Could you check a few things on this model? Use its own coordinates, in mm. A direction names the side the tool comes from. Round coordinates to 2 decimals unless told otherwise and drop trailing zeros. Write each loop counter-clockwise with the first axis right and the second up, starting at its lowest first coordinate (ties: lowest second). Pieces come first, ordered by that corner, then holes. Notation, with made-up numbers: (-16.75, 26) -> (-2.75, 26) arc R28 ccw to (-2.75, 63) -> close; hole circle Ø11 at (40.5, 61). An arc over 180 degrees is marked (long way). Return JSON: item names as keys, results as strings.
from build123d import *

# Parameters (mm, degrees)
SKETCH_1_W          = 10
SKETCH_1_H          = 10
SKETCH_1_W_2        = 8
SKETCH_1_H_2        = 8
EXTRUDE_1_DEPTH     = 495
SKETCH_2_R          = 1.6
CUT_EXTRUDE_1_DEPTH = 496.126246527
CUT_EXTRUDE_2_REACH = 497.126
SKETCH_3_R          = 3
SKETCH_8_R          = 1.6
CUT_EXTRUDE_7_DEPTH = 496.126246527


with BuildPart() as part:
    # ｽｹｯﾁ1 → 押し出し-薄板1 (new body)
    with BuildSketch(Plane.XY):
        Rectangle(SKETCH_1_W, SKETCH_1_H)
        Rectangle(SKETCH_1_W_2, SKETCH_1_H_2, mode=Mode.SUBTRACT)
    extrude(amount=EXTRUDE_1_DEPTH)

    # ｽｹｯﾁ2 → ｶｯﾄ - 押し出し1 (cut, through all)
    with BuildSketch(Plane(origin=(0, 5, 0), x_dir=(1, 0, 0), z_dir=(0, 1, 0))):
        with Locations(Location((0, -5, 0), (0, 0, 180))):
            Circle(SKETCH_2_R)
        with Locations(Location((0, -490, 0), (0, 0, 180))):
            Circle(SKETCH_2_R)
        with Locations(Location((0, -470, 0), (0, 0, 180))):
            Circle(SKETCH_2_R)
    extrude(amount=-CUT_EXTRUDE_1_DEPTH, mode=Mode.SUBTRACT)

    # ｽｹｯﾁ3 → ｶｯﾄ - 押し出し2 (cut, up to next)
    with BuildSketch(Plane(origin=(0, 5, 0), x_dir=(1, 0, 0), z_dir=(0, 1, 0)), mode=Mode.PRIVATE) as cut_extrude_2_sk1:
        with Locations(Location((0, -5, 0), (0, 0, 180))):
            Circle(SKETCH_3_R)
    cut_extrude_2_tool1 = extrude(cut_extrude_2_sk1.sketch, amount=-CUT_EXTRUDE_2_REACH, mode=Mode.PRIVATE) & part.part
    # ｽｹｯﾁ3 → ｶｯﾄ - 押し出し2 (cut, up to next)
    with BuildSketch(Plane(origin=(0, 5, 0), x_dir=(1, 0, 0), z_dir=(0, 1, 0)), mode=Mode.PRIVATE) as cut_extrude_2_sk2:
        with Locations(Location((0, -490, 0), (0, 0, 180))):
            Circle(SKETCH_3_R)
    cut_extrude_2_tool2 = extrude(cut_extrude_2_sk2.sketch, amount=-CUT_EXTRUDE_2_REACH, mode=Mode.PRIVATE) & part.part
    # ｽｹｯﾁ3 → ｶｯﾄ - 押し出し2 (cut, up to next)
    with BuildSketch(Plane(origin=(0, 5, 0), x_dir=(1, 0, 0), z_dir=(0, 1, 0)), mode=Mode.PRIVATE) as cut_extrude_2_sk3:
        with Locations(Location((0, -470, 0), (0, 0, 180))):
            Circle(SKETCH_3_R)
    cut_extrude_2_tool3 = extrude(cut_extrude_2_sk3.sketch, amount=-CUT_EXTRUDE_2_REACH, mode=Mode.PRIVATE) & part.part
    add(cut_extrude_2_tool1.solids().sort_by_distance((0, 5, 5))[0], mode=Mode.SUBTRACT)
    add(cut_extrude_2_tool2.solids().sort_by_distance((0, 5, 490))[0], mode=Mode.SUBTRACT)
    add(cut_extrude_2_tool3.solids().sort_by_distance((0, 5, 470))[0], mode=Mode.SUBTRACT)

    # ｽｹｯﾁ8 → ｶｯﾄ - 押し出し7 (cut, through all)
    with BuildSketch(Plane(origin=(5, 0, 0), x_dir=(0, 0, -1), z_dir=(1, 0, 0))):
        with Locations(Location((-490, 0, 0), (0, 0, 90))):
            Circle(SKETCH_8_R)
        with Locations(Location((-475, 0, 0), (0, 0, 90))):
            Circle(SKETCH_8_R)
    extrude(amount=-CUT_EXTRUDE_7_DEPTH, mode=Mode.SUBTRACT)


solid = part.part
1) I want a section at A-A, the plane y = 0. Please give me the cut outline in (x, z).
Return value:
{"outline": "(-5, 0) -> (-4, 0) -> (-4, 473.4) -> (-5, 473.4) -> close; (-5, 476.6) -> (-4, 476.6) -> (-4, 488.4) -> (-5, 488.4) -> close; (-5, 491.6) -> (-4, 491.6) -> (-4, 495) -> (-5, 495) -> close; (4, 0) -> (5, 0) -> (5, 473.4) -> (4, 473.4) -> close; (4, 476.6) -> (5, 476.6) -> (5, 488.4) -> (4, 488.4) -> close; (4, 491.6) -> (5, 491.6) -> (5, 495) -> (4, 495) -> close"}
2) I want a section at B-B, the plane z = 440. Please give me the cut outline in (x, y).
Return value:
{"outline": "(-5, -5) -> (5, -5) -> (5, 5) -> (-5, 5) -> close; hole (-4, -4) -> (4, -4) -> (4, 4) -> (-4, 4) -> close"}
3) For faces 4 (the face through (0, 4, 244)), 5 (the face through (0, 5, 244)), which set-ups out of +Z, -Z, +X, -X, +Y, -Y let a thin tool reach every point of the face, with its end or its side?
Return value:
{"face 4": "+Z, -Z", "face 5": "+Z, -Z, +X, -X, +Y"}
4) If I drill on probe 1 along Z at (x, y) = (0, -4.8); probe 2 along Z at (x, y) = (-4.25, 0); probe 3 along Z at (x, y) = (0, 4.7), over which ranges is the centre line in solid material (lowest first)? Write a range as [from, to].
Return value:
{"probe 1": "[0, 3.4], [6.6, 468.4], [471.6, 488.4], [491.6, 495]", "probe 2": "[0, 473.4], [476.6, 488.4], [491.6, 495]", "probe 3": "[0, 2], [8, 467], [473, 487], [493, 495]"}
5) Will these pins go through, and if not, where does the flat tip stop? pin 1 Ø3 at (x, z) = (0, 470) entering from +Y; pin 2 Ø5 at (x, z) = (0, 490) entering from +Y.
Return value:
{"pin 1": "through", "pin 2": "y = -4"}
6) Thinking about a two-plate mould opening in Y: for faces 1 (the face through (5, 0, 244)), 2 (the face through (4, 0, 244)), 3 (the face through (0, -5, 244)), which applies, pulls with the +Y half, pulls with the -Y half, needs draft (parallel to the pull), parting line crosses it, or undercut?
Return value:
{"face 1": "needs draft", "face 2": "undercut", "face 3": "pulls with the -Y half"}
